The model under review builds one solid part; all positions refer to its coordinate system, in mm. A direction names the side the tool comes from. Round coordinates to 2 decimals unless told otherwise and drop trailing zeros. Write each loop counter-clockwise with the first axis right and the second up, starting at its lowest first coordinate (ties: lowest second). Pieces come first, ordered by that corner, then holes.
Item 1: Add section B-B (z = 8.5). Give the boundary of the cut face in (x, y) (3 decimals).
Item 2: To check wall thickness, follow L1, parallel to X at y = 3, z = 5.5; L2, parallel to Y at x = 15, z = 3; L3, parallel to X at y = 8, z = 4. State the ranges of each line that lie inside material, in increasing order.
Item 3: Machinability: for faces 4 (the face through (16, 3.513, 4)), 5 (the face through (-16.6, 0.8, 0.3)), 6 (the face through (-17.702, 3.213, 0.285)), 7 (the face through (11.336, 0.77, 5.056)), 8 (the face through (-16.6, 0.8, 9.7)), which of the approach directions +Z, -Z, +X, -X, +Y, -Y give a long, thin tool a straight path to every point of the face, cutting with its end or side? Answer none if there is none.
Item 4: Clearance check with flat-ended pins moving along their axes: pin 1 Ø5 at (y, z) = (13, 7) entering from +X; pin 2 Ø3 at (y, z) = (13, 4) entering from +X; pin 3 Ø4.5 at (x, z) = (16, 4.5) entering from +Y; pin 4 Ø2.5 at (x, z) = (-17.37, 5) entering from -Y. State where each tip first meets the part, or that it passes through.
Item 5: Draft analysis for pull direction X (two halves, no side actions). For faces 1 (the face through (15, 0.513, 5)), 2 (the face through (0.2, 11.1, 4.9)), 3 (the face through (20.79, 0.8, 5.07)), state which applies: +X half, -X half, draft (parallel to the pull), parting line (faces both ways), or undercut.
Item 6: Add section A-A (z = 5). State how many separate pieces and enclosed holes the cut face has, plus the area to 3 significant figures.
```python
from build123d import *

# Parameters (mm, degrees)
BOSS_EXTRUDE1_DEPTH = 10
CUT_EXTRUDE1_REACH  = 27.796
SKETCH2_R           = 1.5
FILLET1_R           = 10
FILLET2_R           = 1


with BuildPart() as part:
    # Sketch1 → Boss-Extrude1 (new body)
    with BuildSketch(Plane.XY):
        with BuildLine():
            Line((-5.459853478, 13), (-5.459853478, 14.5))
            Line((-5.459853478, 14.5), (5.459853478, 14.5))
            Line((5.459853478, 14.5), (5.459853478, 13))
            ThreePointArc((5.459853478, 13), (10.669887711, 9.21756455), (13.655283113, 3.513295191))
            Line((13.655283113, 3.513295191), (21.088125543, 3.513295191))
            Line((21.088125543, 3.513295191), (21.088125543, 0.513295191))
            Line((21.088125543, 0.513295191), (11.088125543, 0.513295191))
            ThreePointArc((11.088125543, 0.513295191), (0, 11.1), (-11.088125543, 0.513295191))
            Line((-11.088125543, 0.513295191), (-21.088125543, 0.513295191))
            Line((-21.088125543, 0.513295191), (-21.088125543, 3.513295191))
            Line((-21.088125543, 3.513295191), (-13.655283113, 3.513295191))
            ThreePointArc((-13.655283113, 3.513295191), (-10.669887711, 9.21756455), (-5.459853478, 13))
        make_face()
    extrude(amount=BOSS_EXTRUDE1_DEPTH)

    # Sketch2 → Cut-Extrude1 (cut, up to next)
    with BuildSketch(Plane(origin=(0, 3.513295191, 0), x_dir=(1, 0, 0), z_dir=(0, 1, 0)), mode=Mode.PRIVATE) as cut_extrude1_sk1:
        with Locations(Location((-17.371704328, -5, 0), (0, 0, 180))):
            Circle(SKETCH2_R)
    cut_extrude1_tool1 = extrude(cut_extrude1_sk1.sketch, amount=-CUT_EXTRUDE1_REACH, mode=Mode.PRIVATE) & part.part
    # Sketch2 → Cut-Extrude1 (cut, up to next)
    with BuildSketch(Plane(origin=(0, 3.513295191, 0), x_dir=(1, 0, 0), z_dir=(0, 1, 0)), mode=Mode.PRIVATE) as cut_extrude1_sk2:
        with Locations(Location((17.371704328, -5, 0), (0, 0, 180))):
            Circle(SKETCH2_R)
    cut_extrude1_tool2 = extrude(cut_extrude1_sk2.sketch, amount=-CUT_EXTRUDE1_REACH, mode=Mode.PRIVATE) & part.part
    add(cut_extrude1_tool1.solids().sort_by_distance((-17.371704, 3.513295, 5))[0], mode=Mode.SUBTRACT)
    add(cut_extrude1_tool2.solids().sort_by_distance((17.371704, 3.513295, 5))[0], mode=Mode.SUBTRACT)

    # Fillet1
    # the kernel refuses this fillet: 10 mm, written as the material it adds along each edge
    with BuildSketch(Plane(origin=(5.459853478, 13, 0), x_dir=(0, 1, 0), z_dir=(0, 0, 1))) as fillet1_piece_1:
        with BuildLine():
            CenterArc((6.552206942, -8.629901796), FILLET1_R, 120.346003633, 23.876636028)
            Line((-1.560741996, -2.783530313), (-1.723000975, -2.666602883))
            ThreePointArc((-1.723000975, -2.666602883), (-0.875816916, -1.338248063), (-0.184397163, 0.07744473))
            Line((-0.184397163, 0.07744473), (0, 0.2))
            ThreePointArc((0, 0.2), (0.75, 0.2), (1.398955861, 0.172598036))
            Line((1.398955861, 0.172598036), (1.5, 0))
        make_face()
    extrude(amount=10)
    with BuildSketch(Plane(origin=(-5.459853478, 13, 0), x_dir=(-0.8722433873059962, -0.4890720532814792, 0), z_dir=(0, 0, 1))) as fillet1_piece_2:
        with BuildLine():
            CenterArc((4.322873472, -9.935762969), FILLET1_R, 96.497751777, 23.876636028)
            Line((-0.73360808, -1.308365081), (-0.834737711, -1.135817123))
            ThreePointArc((-0.834737711, -1.135817123), (-0.541252717, -0.55636813), (-0.174448677, 0.097814411))
            Line((-0.174448677, 0.097814411), (0.022632845, 0.198715259))
            ThreePointArc((0.022632845, 0.198715259), (1.595615601, 0.109425786), (3.168598356, 0.198715259))
            Line((3.168598356, 0.198715259), (3.191231202, 0))
        make_face()
    extrude(amount=10)

    # Fillet2
    fillet2_edges = [part.edges().sort_by_distance(p)[0] for p in [
        (16.088125543, 0.513295191, 0),
        (0, 11.1, 0),
        (11.644446087, 7.950904057, 10),
        (-16.088125543, 0.513295191, 0),
        (-17.371704328, 3.513295191, 0),
        (0, 14.5, 0),
        (11.644446087, 7.950904057, 0),
        (17.371704328, 3.513295191, 0),
        (21.088125543, 0.513295191, 5),
        (11.088125543, 0.513295191, 5),
        (-11.088125543, 0.513295191, 5),
        (0, 14.5, 10),
        (-21.088125543, 0.513295191, 5),
        (-21.088125543, 3.513295191, 5),
        (-13.655283113, 3.513295191, 5),
        (-5.459853478, 14.5, 5),
        (5.459853478, 14.5, 5),
        (13.655283113, 3.513295191, 5),
        (21.088125543, 3.513295191, 5),
        (-17.371704328, 3.513295191, 10),
        (-16.088125543, 0.513295191, 10),
        (-11.644446087, 7.950904057, 0),
        (-11.644446087, 7.950904057, 10),
        (0, 11.1, 10),
        (6.691602977, 12.824105977, 0),
        (6.691602977, 12.824105977, 10),
        (-6.691602977, 12.824105977, 0),
        (-6.691602977, 12.824105977, 10),
        (16.088125543, 0.513295191, 10),
        (17.371704328, 3.513295191, 10),
    ]]
    fillet(fillet2_edges, radius=FILLET2_R)


solid = part.part
```
Numbers:
1. outline: (-21.088, 1.513) arc R1 ccw to (-20.088, 0.513) - (-12.005, 0.513) arc R1 ccw to (-11.013, 1.388) arc R11.1 cw to (11.013, 1.388) arc R1 ccw to (12.005, 0.513) - (20.088, 0.513) arc R1 ccw to (21.088, 1.513) - (21.088, 2.513) arc R1 ccw to (20.088, 3.513) - (14.41, 3.513) arc R1 cw to (13.455, 4.214) arc R14.1 ccw to (8.243, 11.439) arc R10 cw to (5.739, 14.05) arc R1 ccw to (4.904, 14.5) - (-4.904, 14.5) arc R1 ccw to (-5.739, 14.05) arc R10 cw to (-8.243, 11.439) arc R14.1 ccw to (-13.455, 4.214) arc R1 cw to (-14.41, 3.513) - (-20.088, 3.513) arc R1 ccw to (-21.088, 2.513) - close
2. L1: x = -20.96 to -18.79, -15.96 to -10.69, 10.69 to 15.96, 18.79 to 20.96
2. L2: y = 0.51 to 3.51
2. L3: x = -11.61 to -7.69, 7.69 to 11.61
3. face 4: +Z, -Z, +X, +Y
3. face 5: -Z, +X, -X, -Y
3. face 6: -Z, -X, +Y
3. face 7: +Z, -Z, -Y
3. face 8: +Z, +X, -X, -Y
4. pin 1: stops at x = 9.41
4. pin 2: stops at x = 8.16
4. pin 3: stops at y = 3.76
4. pin 4: passes through
5. face 1: draft
5. face 2: undercut
5. face 3: +X half
6. separate pieces: 3
6. enclosed holes: 0
6. area: 150 mm2
